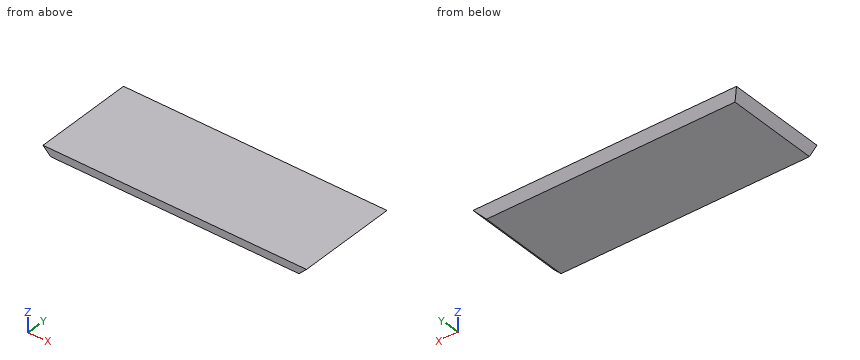
```python
from build123d import *

# Parameters (mm, degrees)
F1_DEPTH = 254
F2_SIZE  = 19.04999


# Not quite as in the source:
# - a fillet or chamfer is up to 0.001 mm smaller than in the source, because OpenCascade refuses the exact size


with BuildPart() as f1:
    # F0 (on Front) → F1 (new body)
    with BuildSketch(Plane.XZ):
        Polygon((333.375, 9.525), (-333.375, 9.525), (-314.325, -9.525), (314.325, -9.525), align=None)
    extrude(amount=-F1_DEPTH)

    # F2 (size 19.05 in the source; OpenCascade refuses exactly that, so slightly less here)
    f2_edges = [f1.edges().sort_by_distance(p)[0] for p in [
        (0, 254, -9.525),
    ]]
    chamfer(f2_edges, length=F2_SIZE)


solid = f1.part
```
Geometry check sheet. Reference: the model listing, model coordinates, mm. Give positions to 0.01 mm unless a question says otherwise; leave off trailing zeros. Write each loop counter-clockwise with the first axis right and the second up, starting at its lowest first coordinate (ties: lowest second). Pieces come first, ordered by that corner, then holes. Notation, with made-up numbers: (76, 45) -> (97, 45) arc R23 cw to (97, 69) -> close; hole circle Ø4 at (87, 69.5). An arc over 180 degrees is marked (long way). Use one line per item in the form item = value.
Item 1: Scan lines: line 1 (Y direction, x = -261, z = 6); line 2 (X direction, y = 31, z = -6); line 3 (X direction, y = 186.5, z = -4). Record each from-to range of solid material in increasing order.
Results list:
line_1 = 0 to 250.48
line_2 = -317.85 to 317.85
line_3 = -319.85 to 319.85
Item 2: Sectioned sample at C-C on z = 5.75. Enter the section's corners in (x, y) (3 decimals), plus the area to 3 significant figures.
Results list:
outline = (-329.6, 0) -> (329.6, 0) -> (329.6, 250.225) -> (-329.6, 250.225) -> close
area = 165,000 mm2
Item 3: Sectioned sample at B-B on y = 45.5. Enter the section's corners in (x, z) (3 decimals), plus the area to 3 significant figures.
Results list:
outline = (-333.375, 9.525) -> (-314.325, -9.525) -> (314.325, -9.525) -> (333.375, 9.525) -> close
area = 12,300 mm2
Item 4: Depth check by flat-ended pin: pin 1 Ø8 at (y, z) = (135, -6.5) entering from +X; pin 2 Ø6 at (x, z) = (-102, 7) entering from -Y; pin 3 Ø1 at (y, z) = (47.5, 3) entering from -X; pin 4 Ø2 at (x, z) = (-17.5, -1) entering from +Y (3 decimals). Enter the tip coordinate at first touch or a pass-through.
Results list:
pin_1 = 321.35
pin_2 = 0
pin_3 = -327.35
pin_4 = 244.475
